Design review of the part built by this model. Coordinates are the model's own, in mm. Face numbers are marked on the shaded views. A direction names the side the tool comes from. Give positions to 0.01 mm unless a question says otherwise; leave off trailing zeros. Loops run counter-clockwise (first coordinate to the right, second up) from the corner with the lowest first, then second, coordinate; pieces in that order, holes last. Notation, with made-up numbers: (0.25, 23.25) - (49.25, 23.25) arc R18 ccw to (49.25, 51.25) - close; hole circle Ø7 at (21.5, 88.25). An arc over 180 degrees is marked (long way). Write each question's results on one line, items separated by ' | '.
```python
from build123d import *

# Parameters (mm, degrees)
F1_DEPTH = 50.8
F3_DEPTH = 85.09
F5_DEPTH = 25.4


with BuildPart() as f1:
    # F0 (on Top) → F1 (new body, symmetric)
    with BuildSketch(Plane.XY):
        Polygon((25.4, -38.1), (0, 0), (-25.4, -38.1), align=None)
    extrude(amount=F1_DEPTH, both=True)

    # F2 (on face) → F3 (join)
    with BuildSketch(Plane(origin=(0, 0, 0), x_dir=(-0.5547001962, 0.8320502943, 0), z_dir=(0.8320502943, 0.5547001962, 0))):
        Polygon((-11.0765361257, 18.9624670893), (-32.9725070827, 18.9624670893), (-43.9204925612, 0), (-32.9725070827, -18.9624670893), (-11.0765361257, -18.9624670893), (-0.1285506472, 0), align=None)
    extrude(amount=F3_DEPTH)

    # F4 (on face) → F5 (join)
    with BuildSketch(Plane.XY.offset(18.9624670893)):
        with BuildLine():
            add(Edge.make_bspline(
                [(21.7850599438, -11.1728273332), (24.91196927, -12.324822675), (34.5838238055, -0.3628267994), (49.6700135525, -7.3872989451), (40.5615667196, 12.1756003251), (36.6019703838, -4.1668657612), (17.0137429969, 0.7146759114), (19.5981739455, -10.3671491954), (21.7850599438, -11.1728273332)],
                knots=[0, 0, 0, 0, 0.1980925373, 0.3554361767, 0.5169793381, 0.6684045786, 0.8614587917, 1, 1, 1, 1], degree=3))
        make_face()
    extrude(amount=F5_DEPTH)


solid = f1.part
```
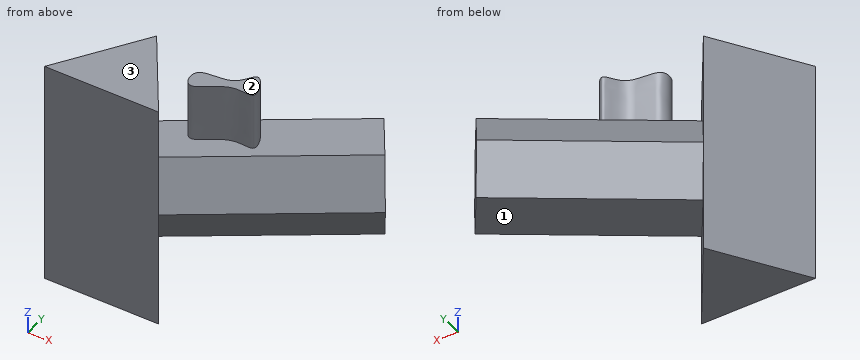
Item 1: We need section D-D on z = 15. Give the boundary of the cut face in (x, y).
Output values:
outline: (-25.4, -38.1) - (25.4, -38.1) - (19.56, -29.34) - (90.36, 17.86) - (75.67, 39.89) - (4.88, -7.31) - (0, 0) - close
Item 2: We need section C-C on x = 16.5. Give the boundary of the cut face in (y, z).
Output values:
outline: (-38.1, -50.8) - (-24.75, -50.8) - (-24.75, -18.96) - (-2.31, -18.96) - (10.85, 0) - (-2.31, 18.96) - (-24.75, 18.96) - (-24.75, 50.8) - (-38.1, 50.8) - close
Item 3: Clearance check with flat-ended pins moving along their axes: P1, Ø9, axis at x = 34.5, y = -3, coming from the +Z side; P2, Ø19.5, axis at x = 29.5, y = 12.5, coming from the +Z side; P3, Ø3, axis at x = 55.5, z = -5, coming from the -Y side. State where each tip first meets the part, or that it passes through.
Output values:
P1: stops at z = 44.36 | P2: stops at z = 18.96 | P3: stops at y = -13.76
Item 4: We need section A-A on z = -10. Give the boundary of the cut face in (x, y).
Output values:
outline: (-25.4, -38.1) - (25.4, -38.1) - (21.16, -31.74) - (91.96, 15.46) - (74.07, 42.29) - (3.27, -4.91) - (0, 0) - close
Item 5: Tool access review of the marked faces 1, 2 and 3: name each direction out of +Z, -Z, +X, -X, +Y, -Y from which nothing blocks a thin tool from reaching the whole face with its end or side.
Output values:
face 1: -Z, +X, +Y | face 2: +Z, +X, +Y | face 3: +Z, +X, -X, +Y, -Y
Item 6: We need section B-B on y = -18.5. Give the boundary of the cut face in (x, z).
Output values:
outline: (-12.33, -50.8) - (12.33, -50.8) - (12.33, -18.96) - (31.69, -18.96) - (51.43, 0) - (31.69, 18.96) - (12.33, 18.96) - (12.33, 50.8) - (-12.33, 50.8) - close
Item 7: Wall thickness on probe 1 along Z at (x, y) = (36, 5); probe 2 along X at (y, z) = (-4, -22.5); probe 3 along X at (y, z) = (31.5, 8.5): over which ranges is each line inside the solid? List them lowest first.
Output values:
probe 1: z = -18.96 to 18.96 | probe 2: x = -2.67 to 2.67 | probe 3: x = 56.33 to 81.27
